Work out the finished part from the listing and answer in its coordinate system (mm). Face numbers are marked on the shaded views. A direction names the side the tool comes from. Round coordinates to 2 decimals unless told otherwise and drop trailing zeros. Write each loop counter-clockwise with the first axis right and the second up, starting at its lowest first coordinate (ties: lowest second). Pieces come first, ordered by that corner, then holes.
1. Find section C-C (z = 12). Write down the section's boundary in (x, y) (3 decimals), and give its area (3 significant figures).
2. Find section B-B (y = 5). Write down the section's boundary in (x, z).
3. Find section A-A (z = 7.5). Write down the section's boundary in (x, y) (3 decimals), and give its area (3 significant figures).
4. Determine the mould class of the marked faces 1, 2 and 3 for opening direction X: pulls with the +X half, pulls with the -X half, needs draft (parallel to the pull), parting line crosses it, or undercut.
5. Flat-ended cylindrical pins translate along their axes: pin 1 Ø11.5 at (x, y) = (1.5, -1.5) entering from +Z; pin 2 Ø12 at (x, z) = (2.5, 16) entering from -Y. Find the tip coordinate at first contact, or state that the pin passes through.
6. Straight lines are drawn through the part: probe 1 along X at (y, z) = (17, 8.5); probe 2 along Z at (x, y) = (-9.5, -3); probe 3 along Y at (x, z) = (13, 27) (3 decimals). For each, find the intervals that lie inside material, in ascending order.
7. A tool of negligible diameter and unlimited length cuts with its end or side. For the marked faces 4 and 5, from which of +Z, -Z, +X, -X, +Y, -Y can it reach the whole face along a straight path? Write none if from no direction.
8. Find section D-D (y = 16.5). Write down the section's boundary in (x, z), and give its area (3 significant figures).
```python
from build123d import *

# Parameters (mm, degrees)
F1_DEPTH = 22.225
F3_DEPTH = 33.02
F4_R     = 8.992991
F5_DEPTH = 33.021


with BuildPart() as f1:
    # F0 (on Front) → F1 (new body, symmetric)
    with BuildSketch(Plane.XZ):
        Polygon((-16.51, 40), (-16.51, 0), (0, 0), (16.51, 0), (16.51, 40), (11.43, 40), (11.43, 5.08), (0, 5.08), (-11.43, 5.08), (-11.43, 40), align=None)
    extrude(amount=F1_DEPTH, both=True)

    # F2 (on face) → F3 (cut)
    with BuildSketch(Plane.YZ.offset(16.51)):
        Polygon((-22.225, 40), (-22.225, 8.714859), (0, 40), align=None)
    extrude(amount=-F3_DEPTH, mode=Mode.SUBTRACT)

    # F4 (on face) → F5 (cut, through all)
    with BuildSketch(Plane.YZ.offset(16.51)):
        with Locations((6.837589, 19.389018)):
            Circle(F4_R)
    extrude(amount=-F5_DEPTH, mode=Mode.SUBTRACT)


solid = f1.part
```
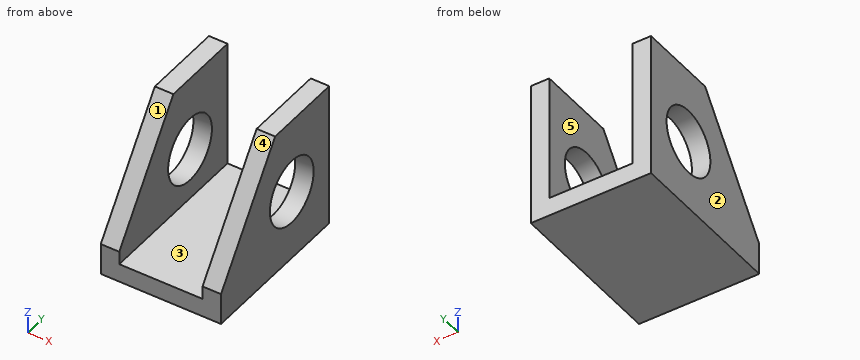
Worked answers:
1. outline: (-16.51, -19.891) - (-11.43, -19.891) - (-11.43, 1.712) - (-16.51, 1.712) - close; (-16.51, 11.964) - (-11.43, 11.964) - (-11.43, 22.225) - (-16.51, 22.225) - close; (11.43, -19.891) - (16.51, -19.891) - (16.51, 1.712) - (11.43, 1.712) - close; (11.43, 11.964) - (16.51, 11.964) - (16.51, 22.225) - (11.43, 22.225) - close
1. area: 324 mm2
2. outline: (-16.51, 0) - (16.51, 0) - (16.51, 10.59) - (11.43, 10.59) - (11.43, 5.08) - (-11.43, 5.08) - (-11.43, 10.59) - (-16.51, 10.59) - close; (-16.51, 28.19) - (-11.43, 28.19) - (-11.43, 40) - (-16.51, 40) - close; (11.43, 28.19) - (16.51, 28.19) - (16.51, 40) - (11.43, 40) - close
3. outline: (-16.51, -22.225) - (-11.43, -22.225) - (-11.43, 22.225) - (-16.51, 22.225) - close; (11.43, -22.225) - (16.51, -22.225) - (16.51, 22.225) - (11.43, 22.225) - close
3. area: 452 mm2
4. face 1: needs draft
4. face 2: pulls with the -X half
4. face 3: undercut
5. pin 1: stops at z = 5.08
5. pin 2: passes through
6. probe 1: x = -16.51 to -11.43, 11.43 to 16.51
6. probe 2: z = 0 to 5.08
6. probe 3: y = -9.235 to 2.047, 11.628 to 22.225
7. face 4: +Z, +X, -X, -Y
7. face 5: +Z, +Y, -Y
8. outline: (-16.51, 0) - (16.51, 0) - (16.51, 40) - (11.43, 40) - (11.43, 5.08) - (-11.43, 5.08) - (-11.43, 40) - (-16.51, 40) - close
8. area: 523 mm2
